```python
from build123d import *

# Parameters (mm, degrees)
F0_W     = 981.075
F0_H     = 44.45
F1_DEPTH = 19.05
F2_W     = 6.35
F2_H     = 11.1125
F3_DEPTH = 981.076
F4_SIZE2 = 3.175
F4_SIZE  = 1.5875
F6_DEPTH = 19.051


with BuildPart() as f1:
    # F0 (on Front) → F1 (new body)
    with BuildSketch(Plane.XZ):
        Rectangle(F0_W, F0_H)
    extrude(amount=F1_DEPTH)

    # F2 (on face) → F3 (cut, through all)
    with BuildSketch(Plane(origin=(-490.5375, 0, 0), x_dir=(0, -1, 0), z_dir=(-1, 0, 0))):
        with Locations((9.525, 16.66875)):
            Rectangle(F2_W, F2_H)
    extrude(amount=-F3_DEPTH, mode=Mode.SUBTRACT)

    # F4
    f4_edges = [f1.edges().sort_by_distance(p)[0] for p in [
        (0, -19.05, 22.225),
    ]]
    chamfer(f4_edges, length=F4_SIZE, length2=F4_SIZE2)

    # F5 (on face) → F6 (cut, through all)
    with BuildSketch(Plane(origin=(0, 0, 0), x_dir=(-1, 0, 0), z_dir=(0, 1, 0))):
        Polygon((-490.5375, 22.225), (-490.5375, -22.225), (-446.0875, 22.225), align=None)
        Polygon((446.0875, 22.225), (490.5375, -22.225), (490.5375, 22.225), align=None)
    extrude(amount=-F6_DEPTH, mode=Mode.SUBTRACT)


solid = f1.part
```
Check sheet for the modelled part. Datum: model origin and axes. Units: mm. Give positions to 0.01 mm unless a question says otherwise; leave off trailing zeros. Write each loop counter-clockwise with the first axis right and the second up, starting at its lowest first coordinate (ties: lowest second). Pieces come first, ordered by that corner, then holes. Notation, with made-up numbers: (54, 20.25) -> (68, 20.25) arc R4 ccw to (68, 27.25) -> close; hole circle Ø5 at (-7, 34.25). An arc over 180 degrees is marked (long way). Use CSV: the item, a comma, the result in double quotes. Start each with the question number.
Q1. Depth check by flat-ended pin: P1, Ø1, axis at y = -16, z = -16, coming from the -X side; P2, Ø4, axis at y = -5, z = 16.5, coming from the -X side; P3, Ø8, axis at y = -10.5, z = -1, coming from the -X side. Enter the tip coordinate at first touch or a pass-through.
Q2. Scan lines: line 1 along Y through (x, z) = (199.5, 16); line 2 along Z through (x, y) = (186.5, -8.5) (1 decimal); line 3 along X through (y, z) = (-12.5, 11). Record each from-to range of solid material in increasing order.
Q3. Cross-section at B-B on z = -14.5. Enter the section's corners in (x, y).
Working result:
1,P1,"stops at x = -484.81"
1,P2,"stops at x = -453.81"
1,P3,"stops at x = -473.31"
2,line 1,"y = -19.05 to -12.7, -6.35 to 0"
2,line 2,"z = -22.2 to 11.1"
2,line 3,"x = -457.31 to 457.31"
3,outline,"(-482.81, -19.05) -> (482.81, -19.05) -> (482.81, 0) -> (-482.81, 0) -> close"
